from build123d import *

# Parameters (mm, degrees)
SKETCH_1_W          = 1960
SKETCH_1_H          = 200
SKETCH_1_R          = 13
EXTRUDE_1566_DEPTH  = 16
SKETCH_2_W          = 1960
SKETCH_2_H          = 16
EXTRUDE_1_DEPTH     = 104
SKETCH_3_R          = 13
CUT_EXTRUDE_1_DEPTH = 1008.372820757


with BuildPart() as part:
    # 草图1 → Extrude 1566 (new body)
    with BuildSketch(Plane.XY):
        with Locations((0, 100)):
            Rectangle(SKETCH_1_W, SKETCH_1_H)
        with Locations((930, 146)):
            Circle(SKETCH_1_R, mode=Mode.SUBTRACT)
        with Locations(Location((-890, 106, 0), (0, 0, 180))):
            Circle(SKETCH_1_R, mode=Mode.SUBTRACT)
        with Locations((850, 146)):
            Circle(SKETCH_1_R, mode=Mode.SUBTRACT)
        with Locations((930, 34)):
            Circle(SKETCH_1_R, mode=Mode.SUBTRACT)
        with Locations((850, 34)):
            Circle(SKETCH_1_R, mode=Mode.SUBTRACT)
        with Locations(Location((-810, 106, 0), (0, 0, 180))):
            Circle(SKETCH_1_R, mode=Mode.SUBTRACT)
        with Locations((770, 34)):
            Circle(SKETCH_1_R, mode=Mode.SUBTRACT)
        with Locations((770, 146)):
            Circle(SKETCH_1_R, mode=Mode.SUBTRACT)
        with Locations(Location((-730, 106, 0), (0, 0, 180))):
            Circle(SKETCH_1_R, mode=Mode.SUBTRACT)
        with Locations((690, 146)):
            Circle(SKETCH_1_R, mode=Mode.SUBTRACT)
        with Locations((690, 34)):
            Circle(SKETCH_1_R, mode=Mode.SUBTRACT)
        with Locations(Location((-650, 106, 0), (0, 0, 180))):
            Circle(SKETCH_1_R, mode=Mode.SUBTRACT)
        with Locations(Location((170, 146, 0), (0, 0, 180))):
            Circle(SKETCH_1_R, mode=Mode.SUBTRACT)
        with Locations(Location((170, 34, 0), (0, 0, 180))):
            Circle(SKETCH_1_R, mode=Mode.SUBTRACT)
        with Locations(Location((-410, 146, 0), (0, 0, 180))):
            Circle(SKETCH_1_R, mode=Mode.SUBTRACT)
        with Locations(Location((250, 34, 0), (0, 0, 180))):
            Circle(SKETCH_1_R, mode=Mode.SUBTRACT)
        with Locations(Location((250, 146, 0), (0, 0, 180))):
            Circle(SKETCH_1_R, mode=Mode.SUBTRACT)
        with Locations(Location((-450, 106, 0), (0, 0, 180))):
            Circle(SKETCH_1_R, mode=Mode.SUBTRACT)
        with Locations(Location((330, 34, 0), (0, 0, 180))):
            Circle(SKETCH_1_R, mode=Mode.SUBTRACT)
        with Locations(Location((330, 146, 0), (0, 0, 180))):
            Circle(SKETCH_1_R, mode=Mode.SUBTRACT)
        with Locations(Location((-370, 106, 0), (0, 0, 180))):
            Circle(SKETCH_1_R, mode=Mode.SUBTRACT)
        with Locations(Location((-290, 106, 0), (0, 0, 180))):
            Circle(SKETCH_1_R, mode=Mode.SUBTRACT)
        with Locations(Location((-210, 106, 0), (0, 0, 180))):
            Circle(SKETCH_1_R, mode=Mode.SUBTRACT)
        with Locations((890, 106)):
            Circle(SKETCH_1_R, mode=Mode.SUBTRACT)
        with Locations((810, 106)):
            Circle(SKETCH_1_R, mode=Mode.SUBTRACT)
        with Locations((650, 106)):
            Circle(SKETCH_1_R, mode=Mode.SUBTRACT)
        with Locations((730, 106)):
            Circle(SKETCH_1_R, mode=Mode.SUBTRACT)
        with Locations((-330, 146)):
            Circle(SKETCH_1_R, mode=Mode.SUBTRACT)
        with Locations((-330, 34)):
            Circle(SKETCH_1_R, mode=Mode.SUBTRACT)
        with Locations((410, 146)):
            Circle(SKETCH_1_R, mode=Mode.SUBTRACT)
        with Locations((-250, 146)):
            Circle(SKETCH_1_R, mode=Mode.SUBTRACT)
        with Locations((-250, 34)):
            Circle(SKETCH_1_R, mode=Mode.SUBTRACT)
        with Locations((450, 106)):
            Circle(SKETCH_1_R, mode=Mode.SUBTRACT)
        with Locations((-170, 34)):
            Circle(SKETCH_1_R, mode=Mode.SUBTRACT)
        with Locations((-170, 146)):
            Circle(SKETCH_1_R, mode=Mode.SUBTRACT)
        with Locations((370, 106)):
            Circle(SKETCH_1_R, mode=Mode.SUBTRACT)
        with Locations(Location((-690, 146, 0), (0, 0, 180))):
            Circle(SKETCH_1_R, mode=Mode.SUBTRACT)
        with Locations((290, 106)):
            Circle(SKETCH_1_R, mode=Mode.SUBTRACT)
        with Locations(Location((-770, 146, 0), (0, 0, 180))):
            Circle(SKETCH_1_R, mode=Mode.SUBTRACT)
        with Locations((210, 106)):
            Circle(SKETCH_1_R, mode=Mode.SUBTRACT)
        with Locations(Location((-850, 146, 0), (0, 0, 180))):
            Circle(SKETCH_1_R, mode=Mode.SUBTRACT)
        with Locations((130, 106)):
            Circle(SKETCH_1_R, mode=Mode.SUBTRACT)
        with Locations(Location((-930, 146, 0), (0, 0, 180))):
            Circle(SKETCH_1_R, mode=Mode.SUBTRACT)
        with Locations(Location((-690, 34, 0), (0, 0, 180))):
            Circle(SKETCH_1_R, mode=Mode.SUBTRACT)
        with Locations(Location((-770, 34, 0), (0, 0, 180))):
            Circle(SKETCH_1_R, mode=Mode.SUBTRACT)
        with Locations(Location((-850, 34, 0), (0, 0, 180))):
            Circle(SKETCH_1_R, mode=Mode.SUBTRACT)
        with Locations(Location((-930, 34, 0), (0, 0, 180))):
            Circle(SKETCH_1_R, mode=Mode.SUBTRACT)
        with Locations(Location((-130, 106, 0), (0, 0, 180))):
            Circle(SKETCH_1_R, mode=Mode.SUBTRACT)
        with Locations((410, 34)):
            Circle(SKETCH_1_R, mode=Mode.SUBTRACT)
        with Locations(Location((-410, 34, 0), (0, 0, 180))):
            Circle(SKETCH_1_R, mode=Mode.SUBTRACT)
    extrude(amount=EXTRUDE_1566_DEPTH)

    # 草图2 → 凸台-拉伸1 (add)
    with BuildSketch(Plane.XY.offset(16)):
        with Locations((0, 192)):
            Rectangle(SKETCH_2_W, SKETCH_2_H)
    extrude(amount=EXTRUDE_1_DEPTH)

    # 草图3 → 切除-拉伸1 (cut, through all)
    with BuildSketch(Plane(origin=(0, 200, 0), x_dir=(-1, 0, 0), z_dir=(0, 1, 0))):
        with Locations(Location((-930, 48, 0), (0, 0, 90))):
            Circle(SKETCH_3_R)
        with Locations(Location((-850, 48, 0), (0, 0, 90))):
            Circle(SKETCH_3_R)
        with Locations(Location((-770, 48, 0), (0, 0, 90))):
            Circle(SKETCH_3_R)
        with Locations(Location((-690, 48, 0), (0, 0, 90))):
            Circle(SKETCH_3_R)
        with Locations(Location((-330, 48, 0), (0, 0, 90))):
            Circle(SKETCH_3_R)
        with Locations(Location((-250, 48, 0), (0, 0, 90))):
            Circle(SKETCH_3_R)
        with Locations(Location((-170, 48, 0), (0, 0, 90))):
            Circle(SKETCH_3_R)
        with Locations(Location((170, 48, 0), (0, 0, 90))):
            Circle(SKETCH_3_R)
        with Locations(Location((250, 48, 0), (0, 0, 90))):
            Circle(SKETCH_3_R)
        with Locations(Location((330, 48, 0), (0, 0, 90))):
            Circle(SKETCH_3_R)
        with Locations(Location((930, 48, 0), (0, 0, 90))):
            Circle(SKETCH_3_R)
        with Locations(Location((850, 48, 0), (0, 0, 90))):
            Circle(SKETCH_3_R)
        with Locations(Location((770, 48, 0), (0, 0, 90))):
            Circle(SKETCH_3_R)
        with Locations(Location((690, 48, 0), (0, 0, 90))):
            Circle(SKETCH_3_R)
        Polygon((-980, 100), (-830, 120), (-980, 120), align=None)
        Polygon((980, 100), (830, 120), (980, 120), align=None)
    extrude(amount=-CUT_EXTRUDE_1_DEPTH, mode=Mode.SUBTRACT)


solid = part.part
Could you check a few things on this model? Use its own coordinates, in mm. A direction names the side the tool comes from. Give positions to 0.01 mm unless a question says otherwise; leave off trailing zeros. Order: outer loops, then holes, each group sorted by start corner. A loop starts at its lowest first (then second) coordinate and runs counter-clockwise, first axis right, second up. Notation, with made-up numbers: (69, -35) -> (84, -35) arc R29 cw to (84, -5) -> close; hole circle Ø5 at (-27, 22). An arc over 180 degrees is marked (long way). Answer in a Markdown table with one row per item. Add a question column.
Item 1: Please list where these lines run through material, in increasing order: probe 1 along Y at (x, z) = (-330, 11.5); probe 2 along Z at (x, y) = (690, 188.5); probe 3 along Y at (x, z) = (-290, 10.5).
Item 2: I'm going to push flat-ended pins straight in: P1, Ø3, axis at x = -637.5, z = 107.5, coming from the -Y side; P2, Ø3, axis at x = -571, y = 156, coming from the +Z side. Where does each tip first touch, or does it pass through?
Item 3: Imagine slicing it at A-A (y = 69). List the corners of the cut face in (x, z) for me, and give its area (3 significant figures).
Item 4: For faces 1 (the flat face through (-14, 93, 16)), 2 (the flat face through (980, 129, 13)), which set-ups out of +Z, -Z, +X, -X, +Y, -Y let a thin tool reach every point of the face, with its end or its side?
Result:
| question | item | result |
|---|---|---|
| 1 | probe 1 | 0 to 21, 47 to 133, 159 to 200 |
| 1 | probe 2 | 0 to 35, 61 to 120 |
| 1 | probe 3 | 0 to 93, 119 to 200 |
| 2 | P1 | y = 184 |
| 2 | P2 | z = 16 |
| 3 | outline | (-980, 0) -> (980, 0) -> (980, 16) -> (-980, 16) -> close |
| 3 | area | 31,400 mm2 |
| 4 | face 1 | +Z, +X, -X, -Y |
| 4 | face 2 | +Z, -Z, +X, +Y, -Y |
